from build123d import *

# Parameters (mm, degrees)
SKETCH1_R           = 9.2
BOSS_EXTRUDE1_DEPTH = 20
CHAMFER1_SIZE       = 3
CHAMFER1_SIZE2      = 4
SKETCH2_R           = 3.3
BOSS_EXTRUDE2_DEPTH = 2
SKETCH3_R           = 1
BOSS_EXTRUDE3_DEPTH = 7.5
CHAMFER2_SIZE       = 0.5
CHAMFER2_SIZE2      = 2.5
SKETCH4_R           = 1
BOSS_EXTRUDE4_DEPTH = 1.5
SKETCH5_R           = 1
BOSS_EXTRUDE5_DEPTH = 15


with BuildPart() as part:
    # Sketch1 → Boss-Extrude1 (new body)
    with BuildSketch(Plane(origin=(0, 0, 0), x_dir=(1, 0, 0), z_dir=(0, 1, 0))):
        with Locations(Location((0, 0, 0), (0, 0, 270))):
            Circle(SKETCH1_R)
    extrude(amount=BOSS_EXTRUDE1_DEPTH)

    # Chamfer1
    chamfer1_edges = [part.edges().sort_by_distance(p)[0] for p in [
        (0, 20, -9.2),
    ]]
    chamfer1_side = [part.faces().sort_by_distance(p)[0] for p in [
        (0, 10, -9.2),
    ]]
    chamfer(chamfer1_edges, length=CHAMFER1_SIZE, length2=CHAMFER1_SIZE2, reference=chamfer1_side[0])

    # Sketch2 → Boss-Extrude2 (add)
    with BuildSketch(Plane(origin=(0, 20, 0), x_dir=(1, 0, 0), z_dir=(0, 1, 0))):
        with Locations(Location((0, 0, 0), (0, 0, 270))):
            Circle(SKETCH2_R)
    extrude(amount=BOSS_EXTRUDE2_DEPTH)

    # Sketch3 → Boss-Extrude3 (add)
    with BuildSketch(Plane(origin=(0, 22, 0), x_dir=(1, 0, 0), z_dir=(0, 1, 0))):
        with Locations(Location((0, 0, 0), (0, 0, 270))):
            Circle(SKETCH3_R)
    extrude(amount=BOSS_EXTRUDE3_DEPTH)

    # Chamfer2
    chamfer2_edges = [part.edges().sort_by_distance(p)[0] for p in [
        (0, 0, -9.2),
    ]]
    chamfer2_side = [part.faces().sort_by_distance(p)[0] for p in [
        (0, 0, 0),
    ]]
    chamfer(chamfer2_edges, length=CHAMFER2_SIZE, length2=CHAMFER2_SIZE2, reference=chamfer2_side[0])

    # Sketch4 → Boss-Extrude4 (add)
    with BuildSketch(Plane.XZ):
        with BuildLine():
            Line((-2.75, 2.75), (-2.75, 13))
            ThreePointArc((-2.75, 13), (0, 15.75), (2.75, 13))
            Line((2.75, 13), (2.75, 2.75))
            Line((2.75, 2.75), (13, 2.75))
            ThreePointArc((13, 2.75), (15.75, 0), (13, -2.75))
            Line((13, -2.75), (2.75, -2.75))
            Line((2.75, -2.75), (2.75, -13))
            ThreePointArc((2.75, -13), (0, -15.75), (-2.75, -13))
            Line((-2.75, -13), (-2.75, -2.75))
            Line((-2.75, -2.75), (-13, -2.75))
            ThreePointArc((-13, -2.75), (-15.75, 0), (-13, 2.75))
            Line((-13, 2.75), (-2.75, 2.75))
        make_face()
        with Locations(Location((0, 13, 0), (0, 0, 270))):
            Circle(SKETCH4_R, mode=Mode.SUBTRACT)
        with Locations(Location((13, 0, 0), (0, 0, 270))):
            Circle(SKETCH4_R, mode=Mode.SUBTRACT)
        with Locations(Location((0, -13, 0), (0, 0, 270))):
            Circle(SKETCH4_R, mode=Mode.SUBTRACT)
        with Locations(Location((-13, 0, 0), (0, 0, 270))):
            Circle(SKETCH4_R, mode=Mode.SUBTRACT)
        with Locations(Location((0, 6.5, 0), (0, 0, 270))):
            Circle(SKETCH4_R, mode=Mode.SUBTRACT)
        with Locations(Location((6.5, 0, 0), (0, 0, 270))):
            Circle(SKETCH4_R, mode=Mode.SUBTRACT)
        with Locations(Location((0, -6.5, 0), (0, 0, 270))):
            Circle(SKETCH4_R, mode=Mode.SUBTRACT)
        with Locations(Location((-6.5, 0, 0), (0, 0, 270))):
            Circle(SKETCH4_R, mode=Mode.SUBTRACT)
    extrude(amount=BOSS_EXTRUDE4_DEPTH)

    # Sketch5 → Boss-Extrude5 (add)
    with BuildSketch(Plane(origin=(0, 0, 0), x_dir=(-0.7071067811865477, 0, -0.7071067811865475), z_dir=(0.7071067811865475, 0, -0.7071067811865477))):
        with Locations(Location((-2.1, 1.25, 0), (0, 0, 330.861265368))):
            Circle(SKETCH5_R)
        with Locations(Location((0, 1.25, 0), (0, 0, 337.716833598))):
            Circle(SKETCH5_R)
        with Locations(Location((2.1, 1.25, 0), (0, 0, 330.024971027))):
            Circle(SKETCH5_R)
    extrude(amount=BOSS_EXTRUDE5_DEPTH)


solid = part.part
Geometry check sheet. Reference: the model listing, model coordinates, mm. A direction names the side the tool comes from. Give positions to 0.01 mm unless a question says otherwise; leave off trailing zeros. Loops run counter-clockwise (first coordinate to the right, second up) from the corner with the lowest first, then second, coordinate; pieces in that order, holes last.
(1) Section check C-C on z = 10. Record the cut outline in (x, y), then the cut area to 3 significant figures.
From the geometry:
outline: (-2.75, -1.5) - (2.75, -1.5) - (2.75, 0) - (-2.75, 0) - close
area: 8.25 mm2
(2) Section check A-A on z = 13.5. Record the cut outline in (x, y), then the cut area to 3 significant figures.
From the geometry:
outline: (-2.7, -1.5) - (-0.87, -1.5) - (-0.87, 0) - (-2.7, 0) - close; (0.87, -1.5) - (2.7, -1.5) - (2.7, 0) - (0.87, 0) - close
area: 5.51 mm2
(3) Section check D-D on z = 0. Count the separate pieces of the cut face and the enclosed holes in it, then the cut area to 3 significant figures.
From the geometry:
separate pieces: 3
enclosed holes: 0
area: 418 mm2
(4) Set-up check for faces 5 (the flat face through (-5, 0, 5)), 6 (the conical face through (-7.746, 0.156, 4.029)), 7 (the cylindrical face through (-0.6, -0.7, -5.7)), 8 (the flat face through (2.75, -1, -8)), 9 (the flat face through (-1.1, 20, 3.4)): record each of +Z, -Z, +X, -X, +Y, -Y from which the full face is reachable in a straight line by a thin tool's end or side.
From the geometry:
face 5: +Z, -X, -Y
face 6: none
face 7: -Y
face 8: -Z, +X, -Y
face 9: +Y
(5) Thickness scan on L1, parallel to X at y = -0.7, z = 0; L2, parallel to Y at x = -2, z = -12.5; L3, parallel to Y at x = -3.5, z = 1. Record the ranges inside material, lowest first.
From the geometry:
L1: x = -15.75 to -14, -12 to -7.5, -5.5 to 5.5, 7.5 to 12, 14 to 15.75
L2: y = -1.5 to 0
L3: y = -1.5 to 20
(6) Depth check by flat-ended pin: pin 1 Ø1.6 at (x, z) = (-6.5, 0) entering from +Y (3 decimals); pin 2 Ø1.7 at (x, z) = (13, 1) entering from +Y; pin 3 Ø1.8 at (x, z) = (0, 6.5) entering from -Y; pin 4 Ø1 at (y, z) = (23.5, -3) entering from -X. Enter the tip coordinate at first touch or a pass-through.
From the geometry:
pin 1: stops at y = 19.625
pin 2: stops at y = 0
pin 3: stops at y = 0
pin 4: passes through
(7) Section check B-B on y = 10. Record the cut outline in (x, z).
From the geometry:
outline: circle Ø18.4 at (0, 0)
(8) Release check for a two-part mould opening along Z. For faces 1 (the flat face through (5, 0, -5)), 2 (the flat face through (0, 0, 6)), 3 (the flat face through (-8, -1, -2.75)), 4 (the cylindrical face through (12, -1, 0)) record: released by +Z, released by -Z, zero draft, split by the parting line, or undercut.
From the geometry:
face 1: zero draft
face 2: undercut
face 3: released by -Z
face 4: undercut
